Source: CAD feature listing. Evaluate the final solid. Frame: model axes, mm. Face numbers are marked on the shaded views. A direction names the side the tool comes from. Coordinates: 2 decimals unless noted, no trailing zeros. Order: outer loops, then holes, each group sorted by start corner. A loop starts at its lowest first (then second) coordinate and runs counter-clockwise, first axis right, second up.
Item 1: Reachability of the marked faces 1 and 2 from +Z, -Z, +X, -X, +Y, -Y: full face, straight path, thin tool, end or side. Return the list, or none.
Item 2: Contact query for flat-ended pins moving along their axis: P1, Ø7.5, axis at x = 25.4, y = 6.35, coming from the -Z side; P2, Ø3, axis at x = 26.5, y = 6.5, coming from the -Z side. Output: stop coordinate, or through.
Item 3: Mould query, pull axis Z, two halves, no side actions, for the marked faces 3, 4 and 5. Classes: released by +Z, released by -Z, zero draft, split by the parting line, or undercut.
Item 4: Section C-C on x = -25.4. Return the cut outline in (y, z) (3 decimals), then the cut area to 3 significant figures.
Item 5: Section B-B on z = -7. Return the cut outline in (x, y) (3 decimals), then the cut area to 3 significant figures.
Item 6: Section D-D on y = 1.75. Return the cut outline in (x, z) (3 decimals), then the cut area to 3 significant figures.
Item 7: Ray query, line 1 (Z direction, x = -2, y = 4.25) (3 decimals); line 2 (Y direction, x = 25.4, z = -9.5) (3 decimals); line 3 (X direction, y = 5.75, z = -7). Return the intervals inside material, ascending.
Item 8: Section A-A on y = 6.35. Return the cut outline in (x, z) (3 decimals), then the cut area to 3 significant figures.
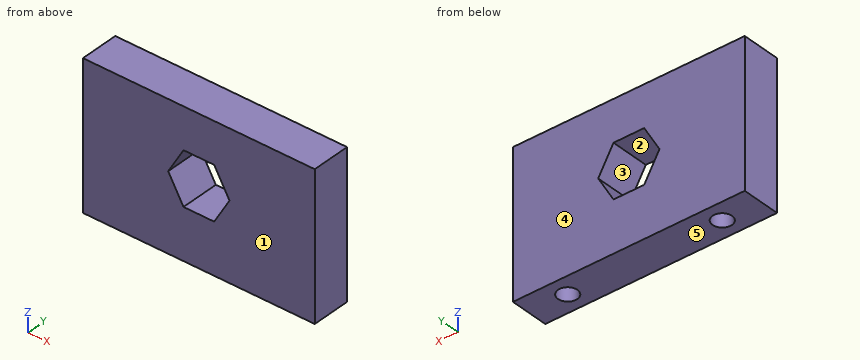
from build123d import *

# Parameters (mm, degrees)
SKETCH1_W           = 76.2
SKETCH1_H           = 47.625
BOSS_EXTRUDE1_DEPTH = 12.7
SKETCH2_R           = 3.175
CUT_EXTRUDE1_DEPTH  = 25.4


with BuildPart() as part:
    # Sketch1 → Boss-Extrude1 (new body)
    with BuildSketch(Plane(origin=(0, 0, 0), x_dir=(1, 0, 0), z_dir=(0, 1, 0))):
        with Locations((0, 1.5875)):
            Rectangle(SKETCH1_W, SKETCH1_H)
        Polygon((10.081979076, 0), (5.040989538, 8.73125), (-5.040989538, 8.73125), (-10.081979076, 0), (-5.040989538, -8.73125), (5.040989538, -8.73125), align=None, mode=Mode.SUBTRACT)
    extrude(amount=BOSS_EXTRUDE1_DEPTH)

    # Sketch2 → Cut-Extrude1 (cut)
    with BuildSketch(Plane(origin=(0, 0, -25.4), x_dir=(-1, 0, 0), z_dir=(0, 0, -1))):
        with Locations((-25.4, 6.35)):
            Circle(SKETCH2_R)
        with Locations((25.4, 6.35)):
            Circle(SKETCH2_R)
    extrude(amount=-CUT_EXTRUDE1_DEPTH, mode=Mode.SUBTRACT)


solid = part.part
Answer list:
1. face 1: +Z, -Z, +X, -X, -Y
1. face 2: +Y, -Y
2. P1: stops at z = -25.4
2. P2: stops at z = 0
3. face 3: undercut
3. face 4: zero draft
3. face 5: released by -Z
4. outline: (0, -25.4) - (3.175, -25.4) - (3.175, 0) - (9.525, 0) - (9.525, -25.4) - (12.7, -25.4) - (12.7, 22.225) - (0, 22.225) - close
4. area: 444 mm2
5. outline: (-38.1, 0) - (-6.041, 0) - (-6.041, 12.7) - (-38.1, 12.7) - close; (6.041, 0) - (38.1, 0) - (38.1, 12.7) - (6.041, 12.7) - close; hole circle Ø6.35 at (-25.4, 6.35); hole circle Ø6.35 at (25.4, 6.35)
5. area: 751 mm2
6. outline: (-38.1, -25.4) - (38.1, -25.4) - (38.1, 22.225) - (-38.1, 22.225) - close; hole (-10.082, 0) - (-5.041, -8.731) - (5.041, -8.731) - (10.082, 0) - (5.041, 8.731) - (-5.041, 8.731) - close
6. area: 3,360 mm2
7. line 1: z = -25.4 to -8.731, 8.731 to 22.225
7. line 2: y = 0 to 3.175, 9.525 to 12.7
7. line 3: x = -38.1 to -28.52, -22.28 to -6.04, 6.04 to 22.28, 28.52 to 38.1
8. outline: (-38.1, -25.4) - (-28.575, -25.4) - (-28.575, 0) - (-22.225, 0) - (-22.225, -25.4) - (22.225, -25.4) - (22.225, 0) - (28.575, 0) - (28.575, -25.4) - (38.1, -25.4) - (38.1, 22.225) - (-38.1, 22.225) - close; hole (-10.082, 0) - (-5.041, -8.731) - (5.041, -8.731) - (10.082, 0) - (5.041, 8.731) - (-5.041, 8.731) - close
8. area: 3,040 mm2
